CAD build for the part. Positions are in the model's coordinates, mm. Face numbers are marked on the shaded views. A direction names the side the tool comes from. Coordinates: 2 decimals unless noted, no trailing zeros. Order: outer loops, then holes, each group sorted by start corner. A loop starts at its lowest first (then second) coordinate and runs counter-clockwise, first axis right, second up.
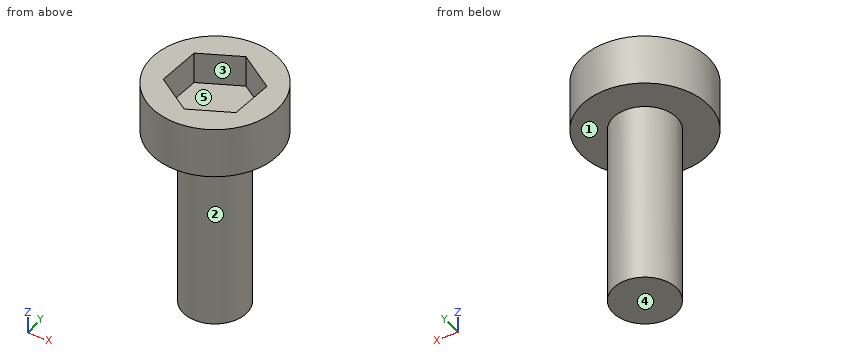
from build123d import *

# Parameters (mm, degrees)
F3_DEPTH = 2.5


with BuildPart() as f1:
    # F0 (on Front) → F1 (revolve)
    with BuildSketch(Plane.XZ):
        Polygon((5.667086, 8.976137), (3.167086, 8.976137), (3.167086, -9.523863), (5.667086, -9.523863), (5.667086, 4.976137), (8.167086, 4.976137), (8.167086, 8.976137), align=None)
    revolve(axis=Axis((3.167086, 0, 1.163182), (0, 0, -1)))

    # F2 (on face) → F3 (cut)
    with BuildSketch(Plane.XY.offset(8.976137)):
        Polygon((2.937124, -3.45646), (6.045487, -1.927383), (6.275449, 1.529077), (3.397048, 3.45646), (0.288685, 1.927383), (0.058723, -1.529077), align=None)
    extrude(amount=-F3_DEPTH, mode=Mode.SUBTRACT)


solid = f1.part
1) Slice it at C-C (z = -7.25). List the corners of the cut face in (x, y), plus the area to 3 significant figures.
2) Two-plate mould, pull along Y, no slides. Class the marked faces 1, 2 and 3: released by +Y, released by -Y, zero draft, split by the parting line, or undercut.
3) Which spindle directions (+Z, -Z, +X, -X, +Y, -Y) get a long thin tool onto all of the face, cutting with end or side? Do the marked faces 4 and 5. Say none if no direction does.
4) Slice it at A-A (x = 4.25). List the corners of the cut face in (y, z).
5) Slice it at B-B (y = 0.25). List the corners of the cut face in (x, z).
6) Slice it at D-D (y = 3.75). List the corners of the cut face in (x, z).
7) Pin check, flat tips, straight feed: P1, Ø1.5, axis at x = 3.5, z = 3, coming from the +Y side; P2, Ø3, axis at y = 2.5, z = 1.5, coming from the +X side. Stop position of each tip, or through.
8) Drill centre lines: probe 1 along Z at (x, y) = (0.25, -3); probe 2 along Z at (x, y) = (2, 1.75); probe 3 along Y at (x, z) = (1.25, -4.5). Where is each one in solid material? Low to high.
Worked out:
1. outline: circle Ø5 at (3.17, 0)
1. area: 19.6 mm2
2. face 1: zero draft
2. face 2: split by the parting line
2. face 3: undercut
3. face 4: -Z, +X, -X, +Y, -Y
3. face 5: +Z
4. outline: (-4.88, 4.98) - (-2.25, 4.98) - (-2.25, -9.52) - (2.25, -9.52) - (2.25, 4.98) - (4.88, 4.98) - (4.88, 8.98) - (2.89, 8.98) - (2.89, 6.48) - (-2.81, 6.48) - (-2.81, 8.98) - (-4.88, 8.98) - close
5. outline: (-1.83, 4.98) - (0.68, 4.98) - (0.68, -9.52) - (5.65, -9.52) - (5.65, 4.98) - (8.16, 4.98) - (8.16, 8.98) - (6.19, 8.98) - (6.19, 6.48) - (0.18, 6.48) - (0.18, 8.98) - (-1.83, 8.98) - close
6. outline: (-0.14, 4.98) - (6.47, 4.98) - (6.47, 8.98) - (-0.14, 8.98) - close
7. P1: stops at y = 2.5
7. P2: stops at x = 5.46
8. probe 1: z = 4.98 to 8.98
8. probe 2: z = -9.52 to 6.48
8. probe 3: y = -1.6 to 1.6
